Could you check a few things on this model? Use its own coordinates, in mm. A direction names the side the tool comes from. Round coordinates to 2 decimals unless told otherwise and drop trailing zeros. Loops run counter-clockwise (first coordinate to the right, second up) from the corner with the lowest first, then second, coordinate; pieces in that order, holes last.
from build123d import *

# Parameters (mm, degrees)
F0_W      = 62
F0_H      = 15
F1_DEPTH  = 1.5
F2_W      = 10
F2_H      = 8
F3_DEPTH  = 1.5
F4_W      = 12
F4_H      = 7
F5_DEPTH  = 1.501
F6_R      = 1.5
F7_DEPTH  = 1.501
F8_W      = 9
F8_H      = 0.5
F9_DEPTH  = 15.001
F10_W     = 2
F10_H     = 1.5
F11_DEPTH = 23.001
F12_W     = 8
F12_H     = 23
F13_DEPTH = 1
F14_R     = 2
F15_R     = 0.5


with BuildPart() as f1:
    # F0 (on Front) → F1 (new body)
    with BuildSketch(Plane.XZ):
        with Locations((-6, 0)):
            Rectangle(F0_W, F0_H)
    extrude(amount=F1_DEPTH)

    # F2 (on face) → F3 (join, through all)
    with BuildSketch(Plane.XZ.offset(1.5)):
        with Locations((20, -11.5)):
            Rectangle(F2_W, F2_H)
    extrude(amount=-F3_DEPTH)

    # F4 (on face) → F5 (cut, through all)
    with BuildSketch(Plane.XZ.offset(1.5)):
        with Locations((-11, -4)):
            Rectangle(F4_W, F4_H)
    extrude(amount=-F5_DEPTH, mode=Mode.SUBTRACT)

    # F6 (on face) → F7 (cut, through all)
    with BuildSketch(Plane.XZ.offset(1.5)):
        with Locations((-32.5, 0)):
            Circle(F6_R)
    extrude(amount=-F7_DEPTH, mode=Mode.SUBTRACT)

    # F8 (on face) → F9 (cut, through all)
    with BuildSketch(Plane(origin=(0, 0, -7.5), x_dir=(1, 0, 0), z_dir=(0, 0, -1))):
        with Locations((-32.5, 1.25)):
            Rectangle(F8_W, F8_H)
    extrude(amount=-F9_DEPTH, mode=Mode.SUBTRACT)

    # F10 (on face) → F11 (cut, through all)
    with BuildSketch(Plane(origin=(0, 0, -15.5), x_dir=(1, 0, 0), z_dir=(0, 0, -1))):
        with Locations((24, 0.75)):
            Rectangle(F10_W, F10_H)
    extrude(amount=-F11_DEPTH, mode=Mode.SUBTRACT)

    # F12 (on face) → F13 (join)
    with BuildSketch(Plane(origin=(0, 0, 0), x_dir=(-1, 0, 0), z_dir=(0, 1, 0))):
        with Locations((-19, -4)):
            Rectangle(F12_W, F12_H)
    extrude(amount=F13_DEPTH)

    # F14
    f14_edges = [f1.edges().sort_by_distance(p)[0] for p in [
        (15, -0.25, -15.5),
        (23, -0.25, -15.5),
        (23, -0.25, 7.5),
        (-5, -0.75, -7.5),
        (-17, -0.75, -7.5),
    ]]
    fillet(f14_edges, radius=F14_R)

    # F15
    f15_edges = [f1.edges().sort_by_distance(p)[0] for p in [
        (23, 1, -4),
        (23, -1.5, -4),
    ]]
    fillet(f15_edges, radius=F15_R)


solid = f1.part
Item 1: Will these pins go through, and if not, where does the flat tip stop? pin 1 (1.2 mm diameter, centred on x = -26.5, y = -0.5, fed in from -Z); pin 2 (4.5 mm diameter, centred on x = -14, z = 3.5, fed in from +Y); pin 3 (10 mm diameter, centred on x = -33.5, z = 0.5, fed in from -Y).
Results list:
pin 1: stops at z = -7.5
pin 2: stops at y = 0
pin 3: stops at y = -1
Item 2: For faces 4 (the flat face through (-28.1, -0.6, -7.5)), 5 (the flat face through (-33, -1, -2)), 6 (the flat face through (-17, -1, -3)), which set-ups out of +Z, -Z, +X, -X, +Y, -Y let a thin tool reach every point of the face, with its end or its side?
Results list:
face 4: -Z, -X, +Y, -Y
face 5: +Z, -Z, -X, -Y
face 6: -Z, +Y, -Y
Item 3: If we section it at C-C, the plane x = 0: Please give me the cut outline in (y, z), then the cut area to 3 significant figures.
Results list:
outline: (-1.5, -7.5) - (0, -7.5) - (0, 7.5) - (-1, 7.5) arc R0.5 ccw to (-1.5, 7) - close
area: 22.4 mm2
Item 4: If I drill on line 1 along Z through (x, y) = (-32.5, -0.15); line 2 along Z through (x, y) = (20, -1.05); line 3 along X through (y, z) = (0.45, -9.5), over which ranges is the centre line in solid material (lowest first)?
Results list:
line 1: z = -7.5 to -1.5, 1.5 to 7.5
line 2: z = -15.5 to 7.5
line 3: x = 15 to 23
Item 5: If we section it at A-A, the plane x = -32.5: Please give me the cut outline in (y, z), then the cut area to 3 significant figures.
Results list:
outline: (-1, -7.5) - (0, -7.5) - (0, -1.5) - (-1, -1.5) - close; (-1, 1.5) - (0, 1.5) - (0, 7.5) - (-1, 7.5) - close
area: 12.0 mm2
Item 6: If we section it at B-B, the plane z = -12.25: Please give me the cut outline in (x, y).
Results list:
outline: (15, -1) arc R0.5 ccw to (15.5, -1.5) - (22.5, -1.5) arc R0.5 ccw to (23, -1) - (23, 0.5) arc R0.5 ccw to (22.5, 1) - (15.5, 1) arc R0.5 ccw to (15, 0.5) - close
Item 7: We'd pull the mould along X, two halves only. Please class faces 1 (the flat face through (-3, -1.5, -1)), 2 (the cylindrical face through (22.43, -0.26, 6.9)), 3 (the cylindrical face through (-17.57, -0.74, -6.9)): released by +X, released by -X, zero draft, split by the parting line, or undercut.
Results list:
face 1: zero draft
face 2: released by +X
face 3: undercut
Item 8: If we section it at D-D, the plane z = 3.5: Please give me the cut outline in (x, y).
Results list:
outline: (-37, -1) - (-28, -1) - (-28, -1.5) - (22.5, -1.5) arc R0.5 ccw to (23, -1) - (23, 0.5) arc R0.5 ccw to (22.5, 1) - (15.5, 1) arc R0.5 ccw to (15, 0.5) - (15, 0) - (-37, 0) - close
